Design review of the part built by this model. Coordinates are the model's own, in mm. A direction names the side the tool comes from. Give positions to 0.01 mm unless a question says otherwise; leave off trailing zeros. Write each loop counter-clockwise with the first axis right and the second up, starting at its lowest first coordinate (ties: lowest second). Pieces come first, ordered by that corner, then holes.
```python
from build123d import *

# Parameters (mm, degrees)
SKETCH1_W           = 45
SKETCH1_H           = 20
BOSS_EXTRUDE2_DEPTH = 12
SKETCH3_R           = 8
CUT_EXTRUDE1_DEPTH  = 51.68530359
CUT_EXTRUDE2_DEPTH  = 4


with BuildPart() as part:
    # Sketch1 → Boss-Extrude2 (new body)
    with BuildSketch(Plane(origin=(0, 0, 0), x_dir=(1, 0, 0), z_dir=(0, 1, 0))):
        with Locations((-22.5, 10)):
            Rectangle(SKETCH1_W, SKETCH1_H)
    extrude(amount=BOSS_EXTRUDE2_DEPTH)

    # Sketch3 → Cut-Extrude1 (cut, through all)
    with BuildSketch(Plane.XZ):
        with Locations(Location((-9.5, -10, 0), (0, 0, 270))):
            Circle(SKETCH3_R)
        with Locations(Location((-35.5, -10, 0), (0, 0, 270))):
            Circle(SKETCH3_R)
    extrude(amount=-CUT_EXTRUDE1_DEPTH, mode=Mode.SUBTRACT)

    # Sketch5 → Cut-Extrude2 (cut)
    with BuildSketch(Plane.XZ):
        with BuildLine():
            Line((-18.140833695, -15.5), (-26.610870323, -15.5))
            ThreePointArc((-26.610870323, -15.5), (-28.107672495, -17.840761906), (-26.359166305, -20))
            Line((-26.359166305, -20), (-18.140833695, -20))
            ThreePointArc((-18.140833695, -20), (-16.55661493, -17.75), (-18.140833695, -15.5))
        make_face()
    extrude(amount=-CUT_EXTRUDE2_DEPTH, mode=Mode.SUBTRACT)


solid = part.part
```
(1) Consider section D-D, the plane z = -18.5. Give the boundary of the cut face in (x, y).
Resolved:
outline: (-45, 0) - (-27.98, 0) - (-27.98, 4) - (-16.68, 4) - (-16.68, 0) - (0, 0) - (0, 12) - (-45, 12) - close
(2) Consider section A-A, the plane z = -10. Give the boundary of the cut face in (x, y), then the cut area to 3 significant figures.
Resolved:
outline: (-45, 0) - (-43.5, 0) - (-43.5, 12) - (-45, 12) - close; (-27.5, 0) - (-17.5, 0) - (-17.5, 12) - (-27.5, 12) - close; (-1.5, 0) - (0, 0) - (0, 12) - (-1.5, 12) - close
area: 156 mm2
(3) Consider section B-B, the plane x = -35.5. Give the boundary of the cut face in (y, z).
Resolved:
outline: (0, -20) - (12, -20) - (12, -18) - (0, -18) - close; (0, -2) - (12, -2) - (12, 0) - (0, 0) - close
(4) To check wall thickness, follow L1, parallel to X at y = 4.5, z = -10; L2, parallel to X at y = 11, z = -12.25; L3, parallel to Z at x = -28.5, y = 4.5. State the ranges of each line that lie inside material, in increasing order.
Resolved:
L1: x = -45 to -43.5, -27.5 to -17.5, -1.5 to 0
L2: x = -45 to -43.18, -27.82 to -17.18, -1.82 to 0
L3: z = -20 to -13.87, -6.13 to 0
(5) Mouldability with a two-part tool opening along Z and no side actions: class faces 3 (the face through (-28.11, 1.97, -17.8)), 4 (the face through (-23, 6, 0)), 5 (the face through (-16.557, 1.972, -17.791)), 6 (the face through (0, 6, -10)) as pulls with the +Z half, pulls with the -Z half, needs draft (parallel to the pull), parting line crosses it, or undercut.
Resolved:
face 3: undercut
face 4: pulls with the +Z half
face 5: undercut
face 6: needs draft
(6) Clearance check with a flat-ended pin moving along its axis: P1, Ø3.5, axis at x = -21.5, z = -18.5, coming from the -Y side. State where the tip first meets the part, or that it passes through.
Resolved:
P1: stops at y = 4
(7) Consider section C-C, the plane y = 3.5. Give the boundary of the cut face in (x, z).
Resolved:
outline: (-45, -20) - (-26.36, -20) arc R2.37 cw to (-26.61, -15.5) - (-18.14, -15.5) arc R2.39 cw to (-18.14, -20) - (0, -20) - (0, 0) - (-45, 0) - close; hole circle Ø16 at (-35.5, -10); hole circle Ø16 at (-9.5, -10)
(8) Tool access review of faces 1 (the face through (-23, 0, -10)), 2 (the face through (-22, 4, -18)): name each direction out of +Z, -Z, +X, -X, +Y, -Y from which nothing blocks a thin tool from reaching the whole face with its end or side.
Resolved:
face 1: +Z, -Z, +X, -X, -Y
face 2: -Y
